Can you work these out from the model? Positions are in its coordinate system, mm. Round coordinates to 2 decimals unless told otherwise and drop trailing zeros. Order: outer loops, then holes, each group sorted by start corner. A loop starts at its lowest first (then second) coordinate and runs counter-clockwise, first axis right, second up.
Q1. If I drill on line 1 (Z direction, x = -52, y = -5); line 2 (Z direction, x = 141, y = -1), over which ranges is the centre line in solid material (lowest first)?
Q2. We'd pull the mould along Z, two halves only. Please class faces 1 (the face through (-11.311, -3.131, 63.785)), 2 (the face through (-23, 0, 52)), 3 (the face through (-249.475, -3.131, 61.705)): pulls with the +Z half, pulls with the -Z half, needs draft (parallel to the pull), parting line crosses it, or undercut.
Q3. If we section it at C-C (x = 149): Please give me the cut outline in (y, z).
Q4. If we section it at A-A (y = -3.5): Please give me the cut outline in (x, z) (3 decimals).
Q5. Will these pins go through, and if not, where does the flat tip stop? P1, Ø7.5, axis at x = -35.87, z = 50.94, coming from the +Y side; P2, Ø3, axis at x = -39.5, y = -4, coming from the +Z side; P3, Ø8, axis at x = 42, z = 65.5, coming from the +Y side.
Q6. If we section it at B-B (z = 60): Please give me the cut outline in (x, y).
from build123d import *

# Parameters (mm, degrees)
F1_DEPTH = 6.35
F3_D     = 6.35


# Not quite as in the source:
# - a length typed as a fraction of an inch, garbled in the dataset ("3 / 203.2 mm" for 3/8 in), is restored


with BuildPart() as f1:
    # F0 (on Front) → F1 (new body)
    with BuildSketch(Plane.XZ):
        Polygon((-242.4979480523, 80.6390420482), (-253.1238703477, 73.6834848906), (-245.7222477886, 49.3858310226), (210.6660933021, 22.1549273185), (213.4919888436, 47.3972393043), align=None)
    extrude(amount=F1_DEPTH)

    # F3 (through all)
    with Locations(Plane.XZ.offset(6.35)):
        with Locations((-35.8659252524, 50.9419701993)):
            Hole(F3_D / 2)


solid = f1.part
Solution:
1. line 1: z = 37.83 to 66.75
1. line 2: z = 26.31 to 52.68
2. face 1: pulls with the +Z half
2. face 2: needs draft
2. face 3: pulls with the -Z half
3. outline: (-6.35, 25.83) - (0, 25.83) - (0, 52.1) - (-6.35, 52.1) - close
4. outline: (-253.124, 73.683) - (-245.722, 49.386) - (210.666, 22.155) - (213.492, 47.397) - (-242.498, 80.639) - close; hole circle Ø6.35 at (-35.866, 50.942)
5. P1: stops at y = 0
5. P2: stops at z = 65.95
5. P3: passes through
6. outline: (-248.96, -6.35) - (40.62, -6.35) - (40.62, 0) - (-248.96, 0) - close
